from build123d import *

# Parameters (mm, degrees)
SKETCH1_R           = 14.2875
BOSS_EXTRUDE1_DEPTH = 76.2
CUT_EXTRUDE1_REACH  = 64.23
SKETCH2_R           = 4.7625
CHAMFER1_SIZE       = 1.5875


with BuildPart() as part:
    # Sketch1 → Boss-Extrude1 (new body)
    with BuildSketch(Plane.XY):
        with BuildLine():
            Line((8.89, 30.48), (-8.89, 30.48))
            ThreePointArc((-8.89, 30.48), (-19.05, -25.4), (31.75, 0))
            ThreePointArc((31.75, 0), (25.4, 19.05), (8.89, 30.48))
        make_face()
        Circle(SKETCH1_R, mode=Mode.SUBTRACT)
    extrude(amount=BOSS_EXTRUDE1_DEPTH)

    # Sketch2 → Cut-Extrude1 (cut, up to next)
    with BuildSketch(Plane(origin=(0, 30.48, 0), x_dir=(1, 0, 0), z_dir=(0, 1, 0)), mode=Mode.PRIVATE) as cut_extrude1_sk1:
        with Locations((0, -57.15)):
            Circle(SKETCH2_R)
    cut_extrude1_tool1 = extrude(cut_extrude1_sk1.sketch, amount=-CUT_EXTRUDE1_REACH, mode=Mode.PRIVATE) & part.part
    add(cut_extrude1_tool1.solids().sort_by_distance((0, 30.48, 57.15))[0], mode=Mode.SUBTRACT)
    # Sketch2 → Cut-Extrude1 (cut, up to next)
    with BuildSketch(Plane(origin=(0, 30.48, 0), x_dir=(1, 0, 0), z_dir=(0, 1, 0)), mode=Mode.PRIVATE) as cut_extrude1_sk2:
        with Locations((0, -19.05)):
            Circle(SKETCH2_R)
    cut_extrude1_tool2 = extrude(cut_extrude1_sk2.sketch, amount=-CUT_EXTRUDE1_REACH, mode=Mode.PRIVATE) & part.part
    add(cut_extrude1_tool2.solids().sort_by_distance((0, 30.48, 19.05))[0], mode=Mode.SUBTRACT)

    # Chamfer1
    chamfer1_edges = [part.edges().sort_by_distance(p)[0] for p in [
        (-14.2875, 0, 0),
        (-14.2875, 0, 76.2),
    ]]
    chamfer(chamfer1_edges, length=CHAMFER1_SIZE)


solid = part.part
Verification items for the finished model (mm, model axes). A direction names the side the tool comes from. Round coordinates to 2 decimals unless told otherwise and drop trailing zeros. Answer in a Markdown table with one row per item. Add a question column.
Q1. Material ranges on line 1 (Z direction, x = 0, y = 19); line 2 (X direction, y = 11.5, z = 6), recorded low to high.
Q2. Section check B-B on x = 0. State how many separate pieces and enclosed holes the cut face has, plus the area to 3 significant figures.
Q3. Tool access check on faces 5 (the face through (-1.03, 22.09, 61.8)), 6 (the face through (-8, -14, 76.2)). Record the directions out of +Z, -Z, +X, -X, +Y, -Y that give a thin tool (end or side, any length) a straight path to the whole face; none if there is none.
Q4. Release check for a two-part mould opening along Y. For faces 1 (the face through (-0.62, 22.09, 14.33)), 2 (the face through (-3.097, -13.948, 37.589)), 3 (the face through (-1.27, -31.725, 37.567)), 4 (the face through (0, 30.48, 38)) record: pulls with the +Y half, pulls with the -Y half, needs draft (parallel to the pull), parting line crosses it, or undercut.
Q5. Gauge pin test, flat ends, axial feed: pin 1 (5 mm diameter, centred on y = -15.5, z = 50.5, fed in from +X); pin 2 (1 mm diameter, centred on y = -9.5, z = 32, fed in from +X); pin 3 (5.5 mm diameter, centred on x = 0, z = 19.05, fed in from +Y). Record the tip position at first contact, or that the pin passes through.
Found:
| question | item | result |
|---|---|---|
| 1 | line 1 | z = 0 to 14.29, 23.81 to 52.39, 61.91 to 76.2 |
| 1 | line 2 | x = -29.59 to -8.48, 8.48 to 29.59 |
| 2 | separate pieces | 4 |
| 2 | enclosed holes | 0 |
| 2 | area | 2,250 mm² |
| 3 | face 5 | +Y |
| 3 | face 6 | +Z, +X, -X, +Y, -Y |
| 4 | face 1 | needs draft |
| 4 | face 2 | undercut |
| 4 | face 3 | parting line crosses it |
| 4 | face 4 | pulls with the +Y half |
| 5 | pin 1 | stops at x = 28.97 |
| 5 | pin 2 | stops at x = 30.45 |
| 5 | pin 3 | stops at y = -14.02 |
